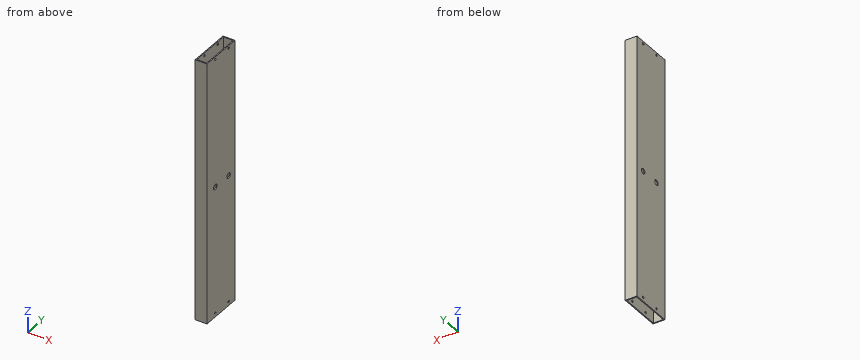
Autodesk Inventor part; units mm, degrees
ref_plane "YZ Plane" through (0, 0, 0) normal (1, 0, 0) x (0, 1, 0)
ref_plane "XZ Plane" through (0, 0, 0) normal (0, 1, 0) x (-1, 0, 0)
ref_plane "XY Plane" through (0, 0, 0) normal (0, 0, 1) x (1, 0, 0)
sketch "Sketch1" plane through (0, 0, 0) normal (0, 0, 1) x (1, 0, 0)
  line L0 (0, 0) -> (18, 0)
  line L1 (18, 0) -> (18, 65)
  line L2 (18, 65) -> (0, 65)
  line L3 (0, 65) -> (0, 0)
  line L4 (1.5, 63.5) -> (16.5, 63.5)
  line L5 (16.5, 63.5) -> (16.5, 1.5)
  line L6 (16.5, 1.5) -> (1.5, 1.5)
  line L7 (1.5, 1.5) -> (1.5, 63.5)
  dimension "d0" = 18
  dimension "d1" = 65
  dimension "d2" = 1.5
extrude "Extrusion1" add sketch "Sketch1" along normal blind 400
sketch "Sketch2" plane through (0, 0, 0) normal (-1, 0, 0) x (0, 0, 1)
  line L0 (0, 65) -> (400, 65)
  circle A0 centre (6, 50.5) radius 1.65
  circle A1 centre (6, 19.5) radius 1.5
  circle A2 centre (396, 19.5) radius 1.65
  circle A3 centre (396, 50.5) radius 1.65
  circle A4 centre (200, 50.5) radius 4
  circle A5 centre (200, 19.5) radius 4
  point P0 (200, 65)
  dimension "d5" = 8
  dimension "d7" = 8
extrude "Extrusion2" cut sketch "Sketch2" against normal blind 20
equation "\"d7\" = d5"
properties part number "X Rail square"
Model file for the job. Use its own axes, mm. Give positions to 0.01 mm unless a question says otherwise; leave off trailing zeros. Order: outer loops, then holes, each group sorted by start corner. A loop starts at its lowest first (then second) coordinate and runs counter-clockwise, first axis right, second up. Notation, with made-up numbers: M 13.5,-38 L 31.5,-38 A28 ccw 31.5,-6 Z; hole C 24,-35.5 d4. An arc over 180 degrees is marked long. Put each result on its own line as item: value. Start each with the question number.
(1) Band-saw the part on C-C on z = 210.5. Give the cut face in (x, y), then the cut area to 3 significant figures.
(2) Band-saw the part on B-B on y = 11.5. Give the cut face in (x, z).
(3) Band-saw the part on A-A on x = 11. Give the cut face in (y, z), then the cut area to 3 significant figures.
(4) Drill centre lines: L1, parallel to Y at x = 17.3, z = 200; L2, parallel to Y at x = 0.4, z = 396; L3, parallel to Y at x = 7.5, z = 149. Where is each one in solid material? Low to high. Write a range as [from, to].
Results below:
1. outline: M 0,0 L 18,0 L 18,65 L 0,65 Z; hole M 1.5,1.5 L 16.5,1.5 L 16.5,63.5 L 1.5,63.5 Z
1. area: 240 mm2
2. outline: M 0,0 L 1.5,0 L 1.5,400 L 0,400 Z; M 16.5,0 L 18,0 L 18,400 L 16.5,400 Z
3. outline: M 0,0 L 1.5,0 L 1.5,400 L 0,400 Z; M 63.5,0 L 65,0 L 65,400 L 63.5,400 Z
3. area: 1,200 mm2
4. L1: y = [0, 15.5], [23.5, 46.5], [54.5, 65]
4. L2: y = [0, 17.85], [21.15, 48.85], [52.15, 65]
4. L3: y = [0, 1.5], [63.5, 65]
